```python
from build123d import *

# Parameters (mm, degrees)
BOSS_EXTRUDE2_DEPTH = 5
SKETCH7_R           = 30
BOSS_EXTRUDE3_DEPTH = 25
SKETCH8_R           = 15
CUT_EXTRUDE2_DEPTH  = 50
BOSS_EXTRUDE4_DEPTH = 9
SKETCH10_R          = 6
CUT_EXTRUDE3_DEPTH  = 9
BOSS_EXTRUDE5_DEPTH = 9
SKETCH12_R          = 6
CUT_EXTRUDE4_DEPTH  = 9


with BuildPart() as part:
    # Sketch6 → Boss-Extrude2 (new body, symmetric)
    with BuildSketch(Plane(origin=(0, 0, 0), x_dir=(1, 0, 0), z_dir=(0, 1, 0))):
        with BuildLine():
            Line((-30, 0), (-122.5, 0))
            Line((-122.5, 0), (-122.5, -15))
            Line((-122.5, -15), (-97.5, -15))
            Line((-97.5, -15), (-4.671688756, -29.634023084))
            ThreePointArc((-4.671688756, -29.634023084), (-22.805160191, -19.491656386), (-30, 0))
        make_face()
    boss_extrude2 = extrude(amount=BOSS_EXTRUDE2_DEPTH, both=True)

    # Sketch7 → Boss-Extrude3 (add, symmetric)
    with BuildSketch(Plane(origin=(0, 0, 0), x_dir=(1, 0, 0), z_dir=(0, 1, 0))):
        with Locations(Location((0, 0, 0), (0, 0, 270))):  # turned: the seam where the file's is
            Circle(SKETCH7_R)
    extrude(amount=BOSS_EXTRUDE3_DEPTH, both=True)

    # Sketch8 → Cut-Extrude2 (cut)
    with BuildSketch(Plane(origin=(0, 25, 0), x_dir=(1, 0, 0), z_dir=(0, 1, 0))):
        with Locations(Location((0, 0, 0), (0, 0, 270))):  # turned: the seam where the file's is
            Circle(SKETCH8_R)
    extrude(amount=-CUT_EXTRUDE2_DEPTH, mode=Mode.SUBTRACT)

    # Mirror1: Boss-Extrude2 across plane
    add(boss_extrude2.mirror(Plane(origin=(0, 5, 0), x_dir=(1, 0, 0), z_dir=(0, 0, -1))))

    # Sketch9 → Boss-Extrude4 (add)
    with BuildSketch(Plane.XY.offset(15)):
        with BuildLine():
            Line((-122.5, 5), (-97.5, 5))
            Line((-97.5, 5), (-97.5, 20))
            ThreePointArc((-97.5, 20), (-110, 32.5), (-122.5, 20))
            Line((-122.5, 20), (-122.5, 5))
        make_face()
    extrude(amount=-BOSS_EXTRUDE4_DEPTH)

    # Sketch10 → Cut-Extrude3 (cut)
    with BuildSketch(Plane.XY.offset(15)):
        with Locations((-110, 20)):
            Circle(SKETCH10_R)
    extrude(amount=-CUT_EXTRUDE3_DEPTH, mode=Mode.SUBTRACT)

    # Sketch11 → Boss-Extrude5 (add)
    with BuildSketch(Plane(origin=(0, 0, -15), x_dir=(-1, 0, 0), z_dir=(0, 0, -1))):
        with BuildLine():
            Line((122.5, 5), (97.5, 5))
            Line((97.5, 5), (97.5, 20))
            ThreePointArc((97.5, 20), (110, 32.5), (122.5, 20))
            Line((122.5, 20), (122.5, 5))
        make_face()
    extrude(amount=-BOSS_EXTRUDE5_DEPTH)

    # Sketch12 → Cut-Extrude4 (cut)
    with BuildSketch(Plane(origin=(0, 0, -15), x_dir=(-1, 0, 0), z_dir=(0, 0, -1))):
        with Locations(Location((110, 20, 0), (0, 0, 180))):  # turned: the seam where the file's is
            Circle(SKETCH12_R)
    extrude(amount=-CUT_EXTRUDE4_DEPTH, mode=Mode.SUBTRACT)


solid = part.part
```
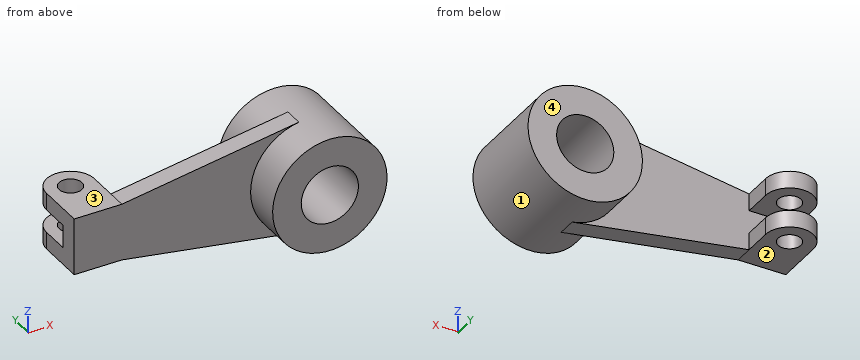
Can you work these out from the model? Positions are in its coordinate system, mm. Face numbers are marked on the shaded views. A direction names the side the tool comes from. Round coordinates to 2 decimals unless told otherwise and drop trailing zeros. Loops run counter-clockwise (first coordinate to the right, second up) from the corner with the lowest first, then second, coordinate; pieces in that order, holes last. Notation, with made-up numbers: (22.5, -40) -> (50.5, -40) arc R12 ccw to (50.5, -31) -> close; hole circle Ø9 at (53.5, 2.25). An arc over 180 degrees is marked (long way). Answer in a Markdown table with one row per item.
Item 1: Will these pins go through, and if not, where does the flat tip stop? P1, Ø4, axis at x = -4, z = 21.5, coming from the +Y side; P2, Ø8, axis at x = -67, z = 7, coming from the +Y side; P3, Ø3, axis at x = -66, y = -6, coming from the +Z side; P4, Ø18, axis at x = 0, z = 0, coming from the -Y side.
Answer block:
| item | result |
|---|---|
| P1 | y = 25 |
| P2 | y = 5 |
| P3 | z = 20.14 |
| P4 | through |
Item 2: If I drill on probe 1 along Z at (x, y) = (-116, 9); probe 2 along X at (y, z) = (-20, 0.5); probe 3 along X at (y, z) = (-3.5, 0.5), over which ranges is the centre line in solid material (lowest first)?
Answer block:
| item | result |
|---|---|
| probe 1 | -15 to -6, 6 to 15 |
| probe 2 | -30 to -14.99, 14.99 to 30 |
| probe 3 | -122.5 to -14.99, 14.99 to 30 |
Item 3: Suppose I cut it at A-A, the plane y = 10.5. List the corners of the cut face in (x, z) for me, plus the area to 3 significant figures.
Answer block:
| item | result |
|---|---|
| outline | (-122.5, -15) -> (-97.5, -15) -> (-97.5, -6) -> (-122.5, -6) -> close; (-122.5, 6) -> (-97.5, 6) -> (-97.5, 15) -> (-122.5, 15) -> close; circle Ø60 at (0, 0); hole circle Ø30 at (0, 0) |
| area | 2,570 mm² |
Item 4: On a 3-axis mill with a long thin cutter (end or side, diameter ignored), from which of +Z, -Z, +X, -X, +Y, -Y can I reach the whole of each face in a straight line? I mean the marked faces 1, 2, 3 and 4. Say none if no direction works.
Answer block:
| item | result |
|---|---|
| face 1 | none |
| face 2 | -Z, -X, +Y, -Y |
| face 3 | +Z, -X, +Y, -Y |
| face 4 | +Z, -Z, +X, +Y |
Item 5: Suppose I cut it at B-B, the plane x = -110. List the corners of the cut face in (y, z) for me.
Answer block:
| item | result |
|---|---|
| outline | (-5, -15) -> (14, -15) -> (14, -6) -> (5, -6) -> (5, 6) -> (14, 6) -> (14, 15) -> (-5, 15) -> close; (26, -15) -> (32.5, -15) -> (32.5, -6) -> (26, -6) -> close; (26, 6) -> (32.5, 6) -> (32.5, 15) -> (26, 15) -> close |
Item 6: Suppose I cut it at D-D, the plane x = 0. List the corners of the cut face in (y, z) for me, plus the area to 3 significant figures.
Answer block:
| item | result |
|---|---|
| outline | (-25, -30) -> (25, -30) -> (25, -15) -> (-25, -15) -> close; (-25, 15) -> (25, 15) -> (25, 30) -> (-25, 30) -> close |
| area | 1,500 mm² |
Item 7: Suppose I cut it at C-C, the plane z = 0. List the corners of the cut face in (x, y) for me.
Answer block:
| item | result |
|---|---|
| outline | (-122.5, -5) -> (-30, -5) -> (-30, -25) -> (-15, -25) -> (-15, 25) -> (-30, 25) -> (-30, 5) -> (-122.5, 5) -> close; (15, -25) -> (30, -25) -> (30, 25) -> (15, 25) -> close |
